Autodesk Fusion 360 part; units mm, degrees
sketch "Sketch1" plane through (0, 0, 0) normal (0, 0, 1) x (1, 0, 0)
  line L0 (2.5647, -2.804) -> (3.7107, 0.819)
  line L1 (3.7107, 0.819) -> (1.146, 3.6231)
  line L2 (1.146, 3.6231) -> (-2.5647, 2.804)
  line L3 (-2.5647, 2.804) -> (-3.7107, -0.819)
  line L4 (-3.7107, -0.819) -> (-1.146, -3.6231)
  line L5 (-1.146, -3.6231) -> (2.5647, -2.804)
  dimension "d1" = 3.8
extrude "Extrude1" add sketch "Sketch1" along normal blind 10
sketch "Sketch2" plane through (0, 0, 10) normal (0, 0, 1) x (-1, 0, 0)
  line L0 (1.146, 3.6231) -> (-2.5647, 2.804)
  line L1 (-2.5647, 2.804) -> (-3.7107, -0.819)
  line L2 (-3.7107, -0.819) -> (-1.146, -3.6231)
  line L3 (-1.146, -3.6231) -> (2.5647, -2.804)
  line L4 (2.5647, -2.804) -> (3.7107, 0.819)
  line L5 (3.7107, 0.819) -> (1.146, 3.6231)
  circle A0 centre (0, 0) radius 0.25
  dimension "d6" = 0.5
extrude "Extrude3" cut sketch "Sketch2" against normal blind 2 contours A0
equation "d1 = polygon_side"
equation "d2 = polygon_height"
equation "polygon_side = 3.8 mm"
equation "polygon_height = 10 mm"
equation "d6 = nail_radius * 2"
equation "nail_radius = 0.25 mm"
equation "nail_depth = 2 mm"
Read the model definition and answer for the solid it produces. Units are mm, in the model's axes. Give positions to 0.01 mm unless a question says otherwise; leave off trailing zeros. Order: outer loops, then holes, each group sorted by start corner. A loop starts at its lowest first (then second) coordinate and runs counter-clockwise, first axis right, second up.
(1) Given pin 1 (2 mm diameter, centred on x = -3, y = 2.5, fed in from -Z); pin 2 (1 mm diameter, centred on y = -1, z = 7.5, fed in from +X); pin 3 (1.5 mm diameter, centred on x = 2, z = 5.5, fed in from +Y), each flat-ended and moving along its own axis, determine where each tip first touches the part or whether it passes through.
(2) Find section D-D (x = -2). Give the vertices of the cut face in (y, z), plus the area to 3 significant figures.
(3) Find section B-B (y = 0). Give the vertices of the cut face in (x, z), plus the area to 3 significant figures.
(4) Find section A-A (z = 7.75). Give the vertices of the cut face in (x, y), plus the area to 3 significant figures.
(5) Find section C-C (x = 0). Give the vertices of the cut face in (y, z).
(6) Straight lines are drawn through the part: L1, parallel to Y at x = 0, z = 9.55; L2, parallel to X at y = 0, z = 8.8; L3, parallel to Y at x = 2.5, z = 9.75. For each, find the intervals that lie inside material, in ascending order.
Result sheet:
1. pin 1: stops at z = 0
1. pin 2: stops at x = 3.29
1. pin 3: stops at y = 3.51
2. outline: (-2.69, 0) - (2.93, 0) - (2.93, 10) - (-2.69, 10) - close
2. area: 56.2 mm2
3. outline: (-3.45, 0) - (3.45, 0) - (3.45, 10) - (0.25, 10) - (0.25, 8) - (-0.25, 8) - (-0.25, 10) - (-3.45, 10) - close
3. area: 68.0 mm2
4. outline: (-3.71, -0.82) - (-1.15, -3.62) - (2.56, -2.8) - (3.71, 0.82) - (1.15, 3.62) - (-2.56, 2.8) - close
4. area: 37.5 mm2
5. outline: (-3.37, 0) - (3.37, 0) - (3.37, 10) - (0.25, 10) - (0.25, 8) - (-0.25, 8) - (-0.25, 10) - (-3.37, 10) - close
6. L1: y = -3.37 to -0.25, 0.25 to 3.37
6. L2: x = -3.45 to -0.25, 0.25 to 3.45
6. L3: y = -2.82 to 2.14
